from build123d import *

# Parameters (mm, degrees)
SKETCH1_W                    = 35
SKETCH1_H                    = 64
BASE_FLANGE1_DEPTH           = 4
EDGE_FLANGE1_STRIP_W         = 17.4732
EDGE_FLANGE1_STRIP_H         = 4
EDGE_FLANGE1_STRIP_CUT_DEPTH = 35
EDGE_FLANGE1_DEPTH           = 35
CUT_EXTRUDE1_DEPTH           = 62.889013565
CUT_EXTRUDE1_DEPTH_BACK      = 62.889013565
SKETCH10_W                   = 20.5
SKETCH10_H                   = 40.5
CUT_EXTRUDE2_DEPTH           = 84.079780934
CUT_EXTRUDE2_DEPTH_BACK      = 84.079780934
SKETCH11_R                   = 4.375
FILLET1_R                    = 17
CUT_EXTRUDE3_DEPTH           = 84.079780934
CUT_EXTRUDE3_DEPTH_BACK      = 84.079780934
CUT_EXTRUDE4_DEPTH           = 58.575624182
CUT_EXTRUDE4_DEPTH_BACK      = 58.575624182
SKETCH14_R                   = 2.1
SKETCH16_R                   = 10.7
CUT_EXTRUDE5_DEPTH           = 0.3
SKETCH21_W                   = 5.45
SKETCH21_H                   = 60
BOSS_EXTRUDE1_DEPTH          = 6
SKETCH23_W                   = 35
SKETCH23_H                   = 2
BOSS_EXTRUDE2_DEPTH          = 10
FILLET2_R                    = 3
FILLET3_R                    = 0.5
FILLET4_R                    = 1
DELETEFACE1_START            = -12.05
DELETEFACE1_DEPTH            = 24.1
MOVE_FACE2_BY                = 1.5
FILLET5_R                    = 0.5
SKETCH26_R                   = 10.7
CUT_EXTRUDE6_DEPTH           = 1.5


# Read off the part's stored shape, not the designer's step: DeleteFace1
# Sheet-metal steps are written as plain solids
with BuildPart() as part:
    # Sketch1 → Base-Flange1 (new body)
    with BuildSketch(Plane.XY):
        Rectangle(SKETCH1_W, SKETCH1_H)
    extrude(amount=-BASE_FLANGE1_DEPTH)

    # Edge-Flange1 strip (across the edge) → Edge-Flange1 strip cut (cut)
    with BuildSketch(Plane(origin=(-17.5, 32, -4), x_dir=(0, -1, 0), z_dir=(1, 0, 0))):
        with Locations((-4, -2)):
            Rectangle(EDGE_FLANGE1_STRIP_W, EDGE_FLANGE1_STRIP_H)
    extrude(amount=EDGE_FLANGE1_STRIP_CUT_DEPTH, mode=Mode.SUBTRACT)

    # Edge-Flange1 section (across the edge) → Edge-Flange1 (add)
    with BuildSketch(Plane(origin=(-17.5, 32, -4), x_dir=(0, -1, 0), z_dir=(1, 0, 0))):
        with BuildLine():
            Line((0, 0.7366), (0, 46))
            Line((0, 46), (4, 46))
            Line((4, 46), (4, 0.7366))
            ThreePointArc((4, 0.7366), (4.215745145, 0.215745145), (4.7366, 0))
            Line((4.7366, 0), (4.7366, -4))
            ThreePointArc((4.7366, -4), (1.38731802, -2.61268198), (0, 0.7366))
        make_face()
    extrude(amount=EDGE_FLANGE1_DEPTH)

    # Sketch10 → Cut-Extrude1 (cut, two sides: drawn at the far end of the back side and taken through both)
    with BuildSketch(Plane.XY.offset(-CUT_EXTRUDE1_DEPTH_BACK)):
        with Locations((0, -2.75)):
            Rectangle(SKETCH10_W, SKETCH10_H)
    extrude(amount=CUT_EXTRUDE1_DEPTH + CUT_EXTRUDE1_DEPTH_BACK, mode=Mode.SUBTRACT)

    # Sketch11 → Cut-Extrude2 (cut, two sides: drawn at the far end of the back side and taken through both)
    with BuildSketch(Plane(origin=(0, 32, 0), x_dir=(1, 0, 0), z_dir=(0, 1, 0)).offset(-CUT_EXTRUDE2_DEPTH_BACK)):
        with Locations(Location((0, 32.5, 0), (0, 0, 270))):
            Circle(SKETCH11_R)
    extrude(amount=CUT_EXTRUDE2_DEPTH + CUT_EXTRUDE2_DEPTH_BACK, mode=Mode.SUBTRACT)

    # Fillet1
    fillet1_edges = [part.edges().sort_by_distance(p)[0] for p in [
        (-17.5, 30, -50),
        (17.5, 30, -50),
    ]]
    fillet(fillet1_edges, radius=FILLET1_R)

    # Sketch13 → Cut-Extrude3 (cut, two sides: drawn at the far end of the back side and taken through both)
    with BuildSketch(Plane(origin=(0, 32, 0), x_dir=(1, 0, 0), z_dir=(0, 1, 0)).offset(-CUT_EXTRUDE3_DEPTH_BACK)):
        with BuildLine():
            Line((12.05, 10), (40.591208969, 10))
            Line((40.591208969, 10), (40.591208969, 59.144369897))
            Line((40.591208969, 59.144369897), (-43.376880173, 59.144369897))
            Line((-43.376880173, 59.144369897), (-43.376880173, 10))
            Line((-43.376880173, 10), (-12.05, 10))
            Line((-12.05, 10), (-12.05, 32.499999826))
            ThreePointArc((-12.05, 32.499999826), (0, 44.55), (12.05, 32.499999826))
            Line((12.05, 32.499999826), (12.05, 10))
        make_face()
    extrude(amount=CUT_EXTRUDE3_DEPTH + CUT_EXTRUDE3_DEPTH_BACK, mode=Mode.SUBTRACT)

    # Sketch14 → Cut-Extrude4 (cut, two sides: drawn at the far end of the back side and taken through both)
    with BuildSketch(Plane.XY.offset(-CUT_EXTRUDE4_DEPTH_BACK)):
        with Locations((-5, 21.75)):
            Circle(SKETCH14_R)
        with Locations((-5, -27.25)):
            Circle(SKETCH14_R)
        with Locations((5, -27.25)):
            Circle(SKETCH14_R)
        with Locations((5, 21.75)):
            Circle(SKETCH14_R)
    extrude(amount=CUT_EXTRUDE4_DEPTH + CUT_EXTRUDE4_DEPTH_BACK, mode=Mode.SUBTRACT)

    # Sketch16 → Cut-Extrude5 (cut)
    with BuildSketch(Plane.XZ.offset(-28)):
        with Locations(Location((0, -32.5, 0), (0, 0, 270))):
            Circle(SKETCH16_R)
    extrude(amount=-CUT_EXTRUDE5_DEPTH, mode=Mode.SUBTRACT)

    # Sketch21 → Boss-Extrude1 (add)
    with BuildSketch(Plane(origin=(0, 0, -4), x_dir=(-1, 0, 0), z_dir=(0, 0, -1))):
        with Locations((-14.775, -2)):
            Rectangle(SKETCH21_W, SKETCH21_H)
        with Locations((14.775, -2)):
            Rectangle(SKETCH21_W, SKETCH21_H)
    extrude(amount=BOSS_EXTRUDE1_DEPTH)

    # Sketch23 → Boss-Extrude2 (add)
    with BuildSketch(Plane(origin=(0, 0, -10), x_dir=(-1, 0, 0), z_dir=(0, 0, -1))):
        with Locations((0, -33)):
            Rectangle(SKETCH23_W, SKETCH23_H)
    extrude(amount=-BOSS_EXTRUDE2_DEPTH)

    # Fillet2
    fillet2_edges = [part.edges().sort_by_distance(p)[0] for p in [
        (-17.5, -34, -5),
        (17.5, -34, -5),
    ]]
    fillet(fillet2_edges, radius=FILLET2_R)

    # Fillet3
    fillet3_edges = [part.edges().sort_by_distance(p)[0] for p in [
        (10.25, 17.5, -2),
        (10.25, -23, -2),
        (-10.25, -23, -2),
        (-10.25, 17.5, -2),
    ]]
    fillet(fillet3_edges, radius=FILLET3_R)

    # Fillet4
    fillet4_edges = [part.edges().sort_by_distance(p)[0] for p in [
        (12.05, -32, -7),
        (-12.05, -32, -7),
    ]]
    fillet(fillet4_edges, radius=FILLET4_R)

    # DeleteFace1 outline → DeleteFace1 (cut)
    with BuildSketch(Plane.YZ.offset(DELETEFACE1_START)):
        with BuildLine():
            ThreePointArc((27.2634, -4), (27.784254855, -4.215745145), (28, -4.7366))
            Line((28, -4.7366), (28, -4))
            Line((28, -4), (27.2634, -4))
        make_face()
    extrude(amount=DELETEFACE1_DEPTH, mode=Mode.SUBTRACT)

    # Move Face2: a face moved outward by 1.5
    extrude(part.faces().sort_by_distance((0, 28, -16.973459017))[0], amount=MOVE_FACE2_BY, dir=(0, -1, 0))

    # Fillet5
    fillet5_edges = [part.edges().sort_by_distance(p)[0] for p in [
        (0, 26.5, -4),
    ]]
    fillet(fillet5_edges, radius=FILLET5_R)

    # Sketch26 → Cut-Extrude6 (cut)
    with BuildSketch(Plane(origin=(0, 32, 0), x_dir=(1, 0, 0), z_dir=(0, 1, 0))):
        with Locations(Location((0, 32.5, 0), (0, 0, 90))):
            Circle(SKETCH26_R)
        with BuildLine():
            Line((-9.05, 22.214694949), (-9.05, 7.7366))
            Line((-9.05, 7.7366), (9.05, 7.7366))
            Line((9.05, 7.7366), (9.05, 22.214694949))
            ThreePointArc((9.05, 22.214694949), (0, 18.8), (-9.05, 22.214694949))
        make_face()
    extrude(amount=-CUT_EXTRUDE6_DEPTH, mode=Mode.SUBTRACT)


solid = part.part
Work out the finished part from the listing and answer in its coordinate system (mm). A direction names the side the tool comes from. Give positions to 0.01 mm unless a question says otherwise; leave off trailing zeros. Write each loop counter-clockwise with the first axis right and the second up, starting at its lowest first coordinate (ties: lowest second). Pieces come first, ordered by that corner, then holes.
Q1. Given pin 1 (13 mm diameter, centred on x = 0, z = -32.5, fed in from +Y); pin 2 (16 mm diameter, centred on x = -1, z = -18, fed in from +Y); pin 3 (1.6 mm diameter, centred on y = 31.5, z = -13.5, fed in from +X); pin 4 (7 mm diameter, centred on x = 5, z = -16, fed in from -Y), each flat-ended and moving along its own axis, determine where each tip first touches the part or whether it passes through.
Answer:
pin 1: stops at y = 30.5
pin 2: stops at y = 32
pin 3: stops at x = 12.05
pin 4: stops at y = 26.5
Q2. The part is cut by section A-A on x = 0. State how many separate pieces and enclosed holes the cut face has, and give its area (3 significant figures).
Answer:
separate pieces: 3
enclosed holes: 0
area: 226 mm2
Q3. The part is cut by section D-D on z = -14.5. Give the vertices of the cut face in (x, y).
Answer:
outline: (-12.05, 26.5) - (12.05, 26.5) - (12.05, 32) - (9.05, 32) - (9.05, 30.5) - (-9.05, 30.5) - (-9.05, 32) - (-12.05, 32) - close
Q4. A tool of negligible diameter and unlimited length cuts with its end or side. For faces 5 (the face through (5, 30.5, -32)), 6 (the face through (-12.05, 29, -21)), 7 (the face through (12.05, -3, -7)), 8 (the face through (-1.68, 29.38, -28.46)), 9 (the face through (6.13, -25.48, -2.03)), from which of +Z, -Z, +X, -X, +Y, -Y can it reach the whole face along a straight path? Write none if from no direction.
Answer:
face 5: +Y
face 6: -Z, -X, +Y, -Y
face 7: -Z
face 8: +Y, -Y
face 9: +Z, -Z
Q5. The part is cut by section C-C on y = -3. Give the vertices of the cut face in (x, z), and give its area (3 significant figures).
Answer:
outline: (-17.5, -10) - (-12.05, -10) - (-12.05, -4) - (-10.25, -4) - (-10.25, 0) - (-17.5, 0) - close; (10.25, -4) - (12.05, -4) - (12.05, -10) - (17.5, -10) - (17.5, 0) - (10.25, 0) - close
area: 123 mm2
Q6. For a pull along X with two mould halves and no side action, classify faces 1 (the face through (0, -23, -2)), 2 (the face through (12.05, 29, -21)), 3 (the face through (-17.5, 0, -5)), 4 (the face through (0, -34, -5)) as released by +X, released by -X, zero draft, split by the parting line, or undercut.
Answer:
face 1: undercut
face 2: released by +X
face 3: released by -X
face 4: zero draft
Q7. The part is cut by section B-B on y = -27.25. Give the vertices of the cut face in (x, z).
Answer:
outline: (-17.5, -10) - (-12.05, -10) - (-12.05, -4) - (-7.1, -4) - (-7.1, 0) - (-17.5, 0) - close; (-2.9, -4) - (2.9, -4) - (2.9, 0) - (-2.9, 0) - close; (7.1, -4) - (12.05, -4) - (12.05, -10) - (17.5, -10) - (17.5, 0) - (7.1, 0) - close
Q8. Straight lines are drawn through the part: L1, parallel to X at y = -27.25, z = -1.6; L2, parallel to Y at x = -5, z = -1.1; L3, parallel to Y at x = -6.5, z = -17. For each, find the intervals that lie inside material, in ascending order.
Answer:
L1: x = -17.5 to -7.1, -2.9 to 2.9, 7.1 to 17.5
L2: y = -34 to -29.35, -25.15 to -23, 17.5 to 19.65, 23.85 to 30.3
L3: y = 26.5 to 30.5
